Check sheet for the drawn part. Datum: minimum x, y, z corner. Units: mm. Round coordinates to 2 decimals unless told otherwise and drop trailing zeros. Write each loop counter-clockwise with the first axis right and the second up, starting at its lowest first coordinate (ties: lowest second). Pieces come first, ordered by that corner, then holes. Notation, with made-up numbers: M 4,31.25 L 26,31.25 A22 cw 26,37.25 Z; hole C -9,-1 d2. An arc over 180 degrees is marked long. Answer in a Markdown table with one row per item. Add a question column.
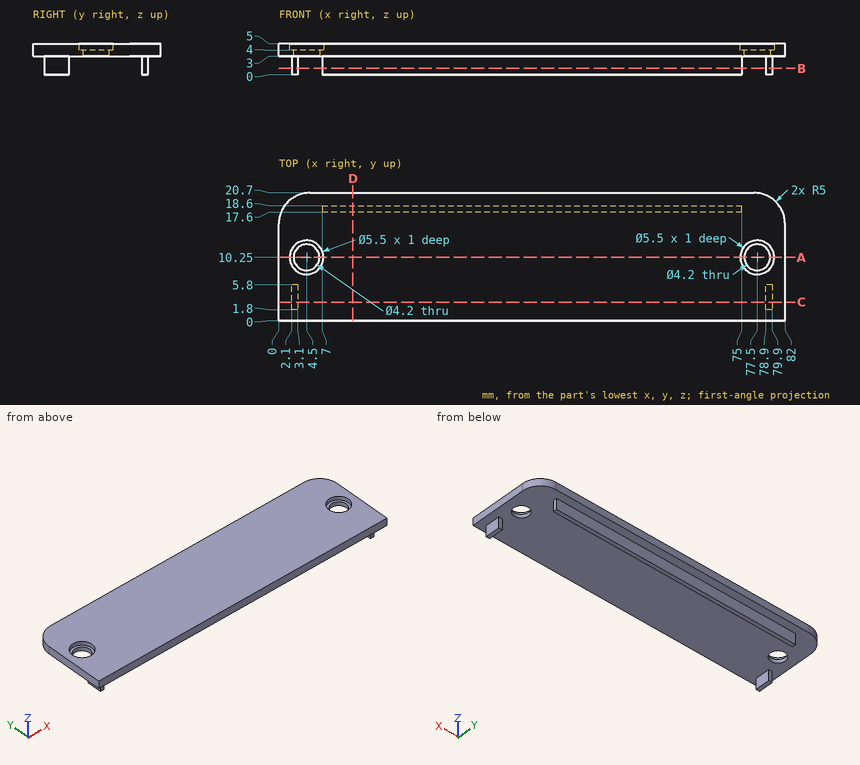
Item 1: Section check D-D, the plane x = 12. Record the boundary of the cut face in (y, z), and give its area (3 significant figures).
Item 2: Scan lines: probe 1 along X at (y, z) = (3.5, 1.05); probe 2 along Z at (x, y) = (22, 16.5); probe 3 along Y at (x, z) = (32, 1.5). Record each from-to range of solid material in increasing order. Write a range as from..to.
Item 3: Section check A-A, the plane y = 10.25. Record the boundary of the cut face in (x, z).
Item 4: Gauge pin test, flat ends, axial feed: pin 1 Ø7 at (x, y) = (4.5, 10.25) entering from -Z; pin 2 Ø1.5 at (y, z) = (4.5, 1) entering from -X; pin 3 Ø0.9 at (x, z) = (35.5, 2) entering from -Y. Record the tip position at first contact, or that the pin passes through.
Item 5: Section check C-C, the plane y = 3. Record the boundary of the cut face in (x, z).
Item 6: Section check B-B, the plane z = 1.05. Record the boundary of the cut face in (x, y), and give its area (3 significant figures).
Result sheet:
| question | item | result |
|---|---|---|
| 1 | outline | M 0,3 L 17.6,3 L 17.6,0 L 18.6,0 L 18.6,3 L 20.7,3 L 20.7,5 L 0,5 Z |
| 1 | area | 44.4 mm^2 |
| 2 | probe 1 | x = 2.1..3.1, 78.9..79.9 |
| 2 | probe 2 | z = 3..5 |
| 2 | probe 3 | y = 17.6..18.6 |
| 3 | outline | M 0,3 L 2.4,3 L 2.4,4 L 1.75,4 L 1.75,5 L 0,5 Z; M 6.6,3 L 75.4,3 L 75.4,4 L 74.75,4 L 74.75,5 L 7.25,5 L 7.25,4 L 6.6,4 Z; M 79.6,3 L 82,3 L 82,5 L 80.25,5 L 80.25,4 L 79.6,4 Z |
| 4 | pin 1 | stops at z = 3 |
| 4 | pin 2 | stops at x = 2.1 |
| 4 | pin 3 | stops at y = 17.6 |
| 5 | outline | M 0,3 L 2.1,3 L 2.1,0 L 3.1,0 L 3.1,3 L 78.9,3 L 78.9,0 L 79.9,0 L 79.9,3 L 82,3 L 82,5 L 0,5 Z |
| 6 | outline | M 2.1,1.8 L 3.1,1.8 L 3.1,5.8 L 2.1,5.8 Z; M 7,17.6 L 75,17.6 L 75,18.6 L 7,18.6 Z; M 78.9,1.8 L 79.9,1.8 L 79.9,5.8 L 78.9,5.8 Z |
| 6 | area | 76.0 mm^2 |
